The listing builds one solid part. Answer for the finished solid, in the listing's coordinates (mm). Face numbers are marked on the shaded views. A direction names the side the tool comes from. Give positions to 0.01 mm unless a question says otherwise; leave off trailing zeros. Loops run counter-clockwise (first coordinate to the right, second up) from the corner with the lowest first, then second, coordinate; pieces in that order, holes last. Notation, with made-up numbers: M -37.75,83 L -20.75,83 A28 cw -20.75,112 Z; hole C -16.5,73 d4. An arc over 180 degrees is marked long. One line per item, written item: value. Start each with the question number.
Q1. A cutting plane is placed at C-C, the plane x = 12.5. Determine the outline of the cut face in (y, z), and give its area (3 significant figures).
Q2. Consider L1, parallel to Y at x = 2.7, z = 2.25; L2, parallel to X at y = -23, z = 11; L3, parallel to Y at x = 0.5, z = 12. Determine where each line is inside the solid, lowest interval first.
Q3. A cutting plane is placed at D-D, the plane y = 20.5. Determine the outline of the cut face in (x, z).
Q4. For the marked faces 1, 2, 3, 4 and 5, determine the directions among +Z, -Z, +X, -X, +Y, -Y from which every point of the face is accessible in a straight line to the end or side of a thin tool.
Q5. The mould has two halves that part along X. Classify the marked faces 6, 7 and 8: +X half, -X half, draft (parallel to the pull), parting line (faces both ways), or undercut.
Q6. Flat-ended cylindrical pins translate along their axes: pin 1 (2 mm diameter, centred on y = -3.5, z = 2, fed in from -X); pin 2 (6 mm diameter, centred on y = -13, z = 11.5, fed in from -X); pin 3 (4 mm diameter, centred on x = 2.5, z = -1, fed in from -Y). Find the tip coordinate at first contact, or state that the pin passes through.
Q7. A cutting plane is placed at B-B, the plane z = -5.5. Determine the outline of the cut face in (x, y), and give its area (3 significant figures).
Q8. A cutting plane is placed at A-A, the plane y = -0.46. State how many separate pieces and enclosed holes the cut face has, and give its area (3 significant figures).
from build123d import *

# Parameters (mm, degrees)
F0_R         = 0.83
F1_DEPTH     = 7
F3_DEPTH     = 20
F0_W         = 6.2750220299
F0_H         = 43
F4_DEPTH     = 25
F5_T         = 2.5
F5_T3_DEPTH  = 6.139113307
F5_T5_DEPTH  = 17.0775900483
F5_T7_DEPTH  = 52.7217752486
F5_T9_DEPTH  = 67.6008063555
F5_T11_DEPTH = 14.360413067
F5_T13_DEPTH = 12.124489639
F5_T15_DEPTH = 6.4792522416
F5_T17_DEPTH = 22.0955071226
F5_T19_DEPTH = 9.4071413577
F5_T21_DEPTH = 34.1892816313
F5_T23_DEPTH = 7.9103027191
F5_T25_DEPTH = 35.7827994693
F5_T27_DEPTH = 54.1950914729
F5_T29_DEPTH = 25.949822152
F5_T31_DEPTH = 35.0076371059
F5_T33_DEPTH = 12.5232163072
F5_T35_DEPTH = 10.1359087229
F5_T37_DEPTH = 18
F6_W         = 12
F6_H         = 12
F7_DEPTH     = 25


# Not quite as in the source:
# - a shell that OpenCascade refuses in one call is made with other operations: the cavity is built on its own and cut out


with BuildPart() as f1:
    # F0 (on Top) → F1 (new body)
    with BuildSketch(Plane.XY):
        Polygon((25, 32.5), (-25, 32.5), (-25, -32.5), (25, -32.5), (25, -23.7771868706), (18.7249779701, -23.7771868706), (18.7249779701, 19.2228131294), (25, 19.2228131294), align=None)
        with Locations((0.16, -3)):
            Circle(F0_R, mode=Mode.SUBTRACT)
        with Locations((2.7, -3)):
            Circle(F0_R, mode=Mode.SUBTRACT)
        with Locations((0.16, -0.46)):
            Circle(F0_R, mode=Mode.SUBTRACT)
        with Locations((2.7, -0.46)):
            Circle(F0_R, mode=Mode.SUBTRACT)
        with Locations((0.16, 2.08)):
            Circle(F0_R, mode=Mode.SUBTRACT)
        with Locations((2.7, 2.08)):
            Circle(F0_R, mode=Mode.SUBTRACT)
    extrude(amount=F1_DEPTH)

    # F2 (on Top) → F3 (join)
    with BuildSketch(Plane.XY):
        Polygon((23.860886693, 31.3004031777), (-23.8608885556, 31.3004031777), (-23.8608885556, -31.3004031777), (-14.5004754886, -31.3004031777), (-14.5004754886, -24.1759135388), (-15.9797277302, -24.1759135388), (-15.9797277302, -7.0804064162), (-20.3868690878, -7.0804064162), (-20.3868690878, 22.1088752151), (-15.9797277302, 22.1088752151), (-15.9797277302, 25.0191779342), (14.8030717392, 25.0191779342), (14.8030717392, -24.1759135388), (-6.1467504129, -24.1759135388), (-6.1467504129, -31.3004031777), (23.860886693, -31.3004031777), align=None)
    extrude(amount=F3_DEPTH)

    # F0 (on Top) → F4 (join)
    with BuildSketch(Plane.XY):
        with Locations((21.8624889851, -2.2771868706)):
            Rectangle(F0_W, F0_H)
    extrude(amount=F4_DEPTH)

    # F5: shell of thickness 2.5, made by hand


with BuildPart() as f5_core1:
    # F5_t2: copy of F1
    add(f1.part)

    # the walls: a layer under each face that stays
    f5_faces = [f5_core1.faces().sort_by_distance(p)[0] for p in [
        (0, 32.5, 3.5),
        (-16.6666666667, 0, 7),
        (1.87, 2.08, 3.5),
        (1.87, -0.46, 3.5),
        (-0.67, 2.08, 3.5),
        (-0.67, -0.46, 3.5),
        (1.87, -3, 3.5),
        (-0.67, -3, 3.5),
        (0, -32.5, 3.5),
        (19.7708149751, -23.7771868706, 22),
        (21.8624889851, -2.2771868706, 25),
        (15.9072574849, -20.8669354518, 20),
        (23.860886693, -27.5387950242, 13.5),
        (8.8570681401, -31.3004031777, 13.5),
        (-6.1467504129, -27.7381583583, 13.5),
        (4.3281606631, -24.1759135388, 13.5),
        (14.8030717392, 0.4216321977, 13.5),
        (-0.5883279955, 25.0191779342, 13.5),
        (-15.9797277302, 23.5640265746, 13.5),
        (-18.183298409, 22.1088752151, 13.5),
        (-20.3868690878, 7.5142343994, 13.5),
        (-18.183298409, -7.0804064162, 13.5),
        (-15.9797277302, -15.6281599775, 13.5),
        (-15.2401016094, -24.1759135388, 13.5),
        (-14.5004754886, -27.7381583583, 13.5),
        (-19.1806820221, -31.3004031777, 13.5),
        (-23.8608885556, 0, 13.5),
        (-9.313e-07, 31.3004031777, 13.5),
        (23.860886693, 25.2616081536, 13.5),
        (23.954162995, 19.2228131294, 22),
        (-16.6666666667, -21.6666666667, 0),
        (-25, 0, 3.5),
        (25, 0, 12.5),
    ]]
    thicken(f5_faces, amount=-F5_T, mode=Mode.SUBTRACT)

    # F5_s4 → F5_t3 (cut)
    with BuildSketch(Plane.YZ.offset(21.360886693)):
        Polygon((19.2478131294, 7.025), (19.2228131294, 4.5), (16.7228131294, 4.5), (16.7228131294, 7), align=None)
        Polygon((-23.8021868706, 7.025), (-23.7771868706, 4.5), (-21.2771868706, 4.5), (-21.2771868706, 7), align=None)
    extrude(amount=F5_T3_DEPTH, mode=Mode.SUBTRACT)

    # F5_s6 → F5_t5 (cut)
    with BuildSketch(Plane.XZ.offset(-33.8004031777)):
        Polygon((23.885886693, 7.025), (23.860886693, 4.5), (21.360886693, 4.5), (21.360886693, 7), align=None)
    extrude(amount=F5_T5_DEPTH, mode=Mode.SUBTRACT)

    # F5_s8 → F5_t7 (cut)
    with BuildSketch(Plane.YZ.offset(-26.3608885556)):
        Polygon((31.3254031777, 7.025), (31.3004031777, 4.5), (28.8004031777, 4.5), (28.8004031777, 7), align=None)
    extrude(amount=F5_T7_DEPTH, mode=Mode.SUBTRACT)

    # F5_s10 → F5_t9 (cut)
    with BuildSketch(Plane.XZ.offset(-33.8004031777)):
        Polygon((-23.8858885556, 7.025), (-23.8608885556, 4.5), (-21.3608885556, 4.5), (-21.3608885556, 7), align=None)
    extrude(amount=F5_T9_DEPTH, mode=Mode.SUBTRACT)

    # F5_s12 → F5_t11 (cut)
    with BuildSketch(Plane.YZ.offset(-26.3608885556)):
        Polygon((-31.3254031777, 7.025), (-31.3004031777, 4.5), (-28.8004031777, 4.5), (-28.8004031777, 7), align=None)
    extrude(amount=F5_T11_DEPTH, mode=Mode.SUBTRACT)

    # F5_s14 → F5_t13 (cut)
    with BuildSketch(Plane.XZ.offset(21.6759135388)):
        Polygon((-14.4754754886, 7.025), (-14.5004754886, 4.5), (-17.0004754886, 4.5), (-17.0004754886, 7), align=None)
        Polygon((-6.1717504129, 7.025), (-6.1467504129, 4.5), (-3.6467504129, 4.5), (-3.6467504129, 7), align=None)
    extrude(amount=F5_T13_DEPTH, mode=Mode.SUBTRACT)

    # F5_s16 → F5_t15 (cut)
    with BuildSketch(Plane.YZ.offset(-18.4797277302)):
        Polygon((-24.1509135388, 7.025), (-24.1759135388, 4.5), (-26.6759135388, 4.5), (-26.6759135388, 7), align=None)
    extrude(amount=F5_T15_DEPTH, mode=Mode.SUBTRACT)

    # F5_s18 → F5_t17 (cut)
    with BuildSketch(Plane.XZ.offset(4.5804064162)):
        Polygon((-15.9547277302, 7.025), (-15.9797277302, 4.5), (-18.4797277302, 4.5), (-18.4797277302, 7), align=None)
    extrude(amount=F5_T17_DEPTH, mode=Mode.SUBTRACT)

    # F5_s20 → F5_t19 (cut)
    with BuildSketch(Plane.YZ.offset(-22.8868690878)):
        Polygon((-7.0554064162, 7.025), (-7.0804064162, 4.5), (-9.5804064162, 4.5), (-9.5804064162, 7), align=None)
        Polygon((22.0838752151, 7.025), (22.1088752151, 4.5), (24.6088752151, 4.5), (24.6088752151, 7), align=None)
    extrude(amount=F5_T19_DEPTH, mode=Mode.SUBTRACT)

    # F5_s22 → F5_t21 (cut)
    with BuildSketch(Plane.XZ.offset(-24.6088752151)):
        Polygon((-20.3618690878, 7.025), (-20.3868690878, 4.5), (-22.8868690878, 4.5), (-22.8868690878, 7), align=None)
    extrude(amount=F5_T21_DEPTH, mode=Mode.SUBTRACT)

    # F5_s24 → F5_t23 (cut)
    with BuildSketch(Plane.XZ.offset(-27.5191779342)):
        Polygon((-15.9547277302, 7.025), (-15.9797277302, 4.5), (-18.4797277302, 4.5), (-18.4797277302, 7), align=None)
    extrude(amount=F5_T23_DEPTH, mode=Mode.SUBTRACT)

    # F5_s26 → F5_t25 (cut)
    with BuildSketch(Plane.YZ.offset(-18.4797277302)):
        Polygon((24.9941779342, 7.025), (25.0191779342, 4.5), (27.5191779342, 4.5), (27.5191779342, 7), align=None)
    extrude(amount=F5_T25_DEPTH, mode=Mode.SUBTRACT)

    # F5_s28 → F5_t27 (cut)
    with BuildSketch(Plane.XZ.offset(-27.5191779342)):
        Polygon((14.7780717392, 7.025), (14.8030717392, 4.5), (17.3030717392, 4.5), (17.3030717392, 7), align=None)
    extrude(amount=F5_T27_DEPTH, mode=Mode.SUBTRACT)

    # F5_s30 → F5_t29 (cut)
    with BuildSketch(Plane.YZ.offset(-8.6467504129)):
        Polygon((-24.1509135388, 7.025), (-24.1759135388, 4.5), (-26.6759135388, 4.5), (-26.6759135388, 7), align=None)
    extrude(amount=F5_T29_DEPTH, mode=Mode.SUBTRACT)

    # F5_s32 → F5_t31 (cut)
    with BuildSketch(Plane.YZ.offset(-8.6467504129)):
        Polygon((-31.3254031777, 7.025), (-31.3004031777, 4.5), (-28.8004031777, 4.5), (-28.8004031777, 7), align=None)
    extrude(amount=F5_T31_DEPTH, mode=Mode.SUBTRACT)

    # F5_s34 → F5_t33 (cut)
    with BuildSketch(Plane.XZ.offset(21.2771868706)):
        Polygon((23.885886693, 7.025), (23.860886693, 4.5), (21.360886693, 4.5), (21.360886693, 7), align=None)
    extrude(amount=F5_T33_DEPTH, mode=Mode.SUBTRACT)

    # F5_s36 → F5_t35 (cut)
    with BuildSketch(Plane.YZ.offset(16.2249779701)):
        Polygon((-23.8021868706, 20.025), (-21.2771868706, 20), (-21.2771868706, 17.5), (-23.7771868706, 17.5), align=None)
        Polygon((19.2478131294, 20.025), (19.2228131294, 17.5), (16.7228131294, 17.5), (16.7228131294, 20), align=None)
    extrude(amount=F5_T35_DEPTH, mode=Mode.SUBTRACT)

    # F5_s38 → F5_t37 (cut)
    with BuildSketch(Plane.XY.offset(4.5)):
        Polygon((23.885886693, -23.8021868706), (23.860886693, -21.2771868706), (21.360886693, -21.2771868706), (21.360886693, -23.7771868706), align=None)
        Polygon((14.7780717392, -24.1509135388), (14.8030717392, -26.6759135388), (17.3030717392, -26.6759135388), (17.3030717392, -24.1759135388), align=None)
        Polygon((14.7780717392, 24.9941779342), (17.3030717392, 25.0191779342), (17.3030717392, 27.5191779342), (14.8030717392, 27.5191779342), align=None)
        Polygon((-15.9547277302, 24.9941779342), (-15.9797277302, 27.5191779342), (-18.4797277302, 27.5191779342), (-18.4797277302, 25.0191779342), align=None)
        Polygon((-20.3618690878, 22.0838752151), (-20.3868690878, 24.6088752151), (-22.8868690878, 24.6088752151), (-22.8868690878, 22.1088752151), align=None)
        Polygon((-20.3618690878, -7.0554064162), (-22.8868690878, -7.0804064162), (-22.8868690878, -9.5804064162), (-20.3868690878, -9.5804064162), align=None)
        Polygon((-15.9547277302, -24.1509135388), (-18.4797277302, -24.1759135388), (-18.4797277302, -26.6759135388), (-15.9797277302, -26.6759135388), align=None)
        Polygon((23.885886693, 19.2478131294), (21.360886693, 19.2228131294), (21.360886693, 16.7228131294), (23.860886693, 16.7228131294), align=None)
    extrude(amount=F5_T37_DEPTH, mode=Mode.SUBTRACT)


with BuildPart() as f1_1:
    add(f1.part)

    # what is left inside the walls is the cavity
    f5_cavity = [f5_core1.part.solids().sort_by_distance(p)[0] for p in [
        (0, -10, 2.525),
    ]]
    add(f5_cavity, mode=Mode.SUBTRACT)

    # F6 (on Top) → F7 (join)
    with BuildSketch(Plane.XY):
        with Locations((-21, 28.5)):
            Rectangle(F6_W, F6_H)
        with Locations((-21, -28.5)):
            Rectangle(F6_W, F6_H)
        with Locations((21, -28.5)):
            Rectangle(F6_W, F6_H)
        with Locations((21, 28.5)):
            Rectangle(F6_W, F6_H)
    extrude(amount=-F7_DEPTH)


solid = f1_1.part
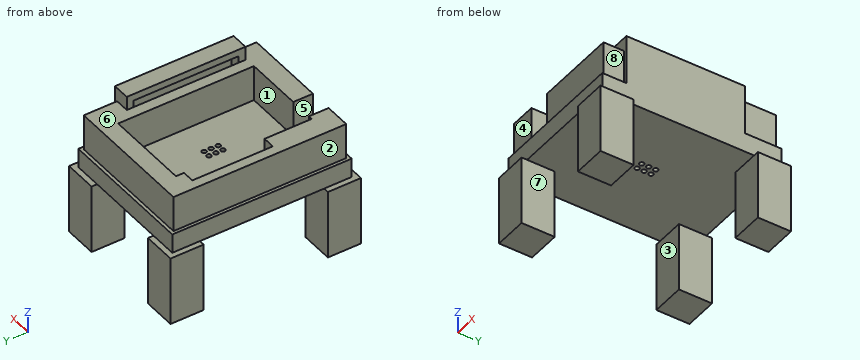
Answer block:
1. outline: M -32.5,0 L 32.5,0 L 32.5,7 L 31.3,7 L 31.3,20 L 25.02,20 L 25.02,7 L -24.18,7 L -24.18,20 L -31.3,20 L -31.3,7 L -32.5,7 Z; hole M -30,2.5 L 30,2.5 L 30,4.5 L 28.8,4.5 L 28.8,17.5 L 27.52,17.5 L 27.52,4.5 L -26.68,4.5 L -26.68,17.5 L -28.8,17.5 L -28.8,4.5 L -30,4.5 Z
1. area: 465 mm^2
2. L1: -32.5 to -3.83, -2.17 to -1.29, 0.37 to 1.25, 2.91 to 32.5
2. L2: -23.86 to -21.36, -18.48 to -15.98, 14.8 to 17.3, 21.36 to 25
2. L3: -31.3 to -28.8, -26.68 to -24.18, 25.02 to 27.52, 28.8 to 31.3
3. outline: M -25,0 L 25,0 L 25,7 L 23.86,7 L 23.86,20 L 14.8,20 L 14.8,7 L -20.39,7 L -20.39,20 L -23.86,20 L -23.86,7 L -25,7 Z; hole M -22.5,2.5 L 22.5,2.5 L 22.5,4.5 L 21.36,4.5 L 21.36,17.5 L 17.3,17.5 L 17.3,4.5 L -22.5,4.5 Z
4. face 1: +Z
4. face 2: +Z, -X, +Y, -Y
4. face 3: -Z, +X, -X
4. face 4: +Z, +X, -X, -Y
4. face 5: +Z, -Y
5. face 6: draft
5. face 7: undercut
5. face 8: +X half
6. pin 1: x = -25
6. pin 2: x = -23.86
6. pin 3: y = -32.5
7. outline: M -27,-34.5 L -15,-34.5 L -15,-22.5 L -27,-22.5 Z; M -27,22.5 L -15,22.5 L -15,34.5 L -27,34.5 Z; M 15,-34.5 L 27,-34.5 L 27,-22.5 L 15,-22.5 Z; M 15,22.5 L 27,22.5 L 27,34.5 L 15,34.5 Z
7. area: 576 mm^2
8. separate pieces: 3
8. enclosed holes: 1
8. area: 378 mm^2
